```python
from build123d import *

# Parameters (mm, degrees)
BOSS_EXTRUDE1_DEPTH = 2
BOSS_EXTRUDE2_DEPTH = 20
FILLET1_R           = 5
CHAMFER1_SIZE       = 3.5
CHAMFER1_SIZE2      = 7.505774222


with BuildPart() as part:
    # Sketch1 → Boss-Extrude1 (new body)
    with BuildSketch(Plane(origin=(0, 0, 0), x_dir=(1, 0, 0), z_dir=(0, 1, 0))):
        with BuildLine():
            ThreePointArc((58.25, 100.891959541), (30.152418754, 112.530358763), (0, 116.5))
            Line((0, 116.5), (0, 105.5))
            ThreePointArc((0, 105.5), (27.305409258, 101.905174673), (52.75, 91.365680099))
            Line((52.75, 91.365680099), (58.25, 100.891959541))
        make_face()
    extrude(amount=BOSS_EXTRUDE1_DEPTH)

    # Sketch1<3> → Boss-Extrude2 (add)
    with BuildSketch(Plane(origin=(0, 0, 0), x_dir=(1, 0, 0), z_dir=(0, 1, 0))):
        with BuildLine():
            ThreePointArc((52.75, 91.365680099), (27.305409258, 101.905174673), (0, 105.5))
            Line((0, 105.5), (0, 101.5))
            ThreePointArc((0, 101.5), (26.270133078, 98.041471368), (50.75, 87.901578484))
            Line((50.75, 87.901578484), (52.75, 91.365680099))
        make_face()
    extrude(amount=BOSS_EXTRUDE2_DEPTH)

    # Fillet1
    fillet1_edges = [part.edges().sort_by_distance(p)[0] for p in [
        (27.305409258, 2, -101.905174673),
    ]]
    fillet(fillet1_edges, radius=FILLET1_R)

    # Chamfer1
    chamfer1_edges = [part.edges().sort_by_distance(p)[0] for p in [
        (27.305409258, 20, -101.905174673),
    ]]
    chamfer1_side = [part.faces().sort_by_distance(p)[0] for p in [
        (26.486113557, 20, -98.847521491),
    ]]
    chamfer(chamfer1_edges, length=CHAMFER1_SIZE, length2=CHAMFER1_SIZE2, reference=chamfer1_side[0])


solid = part.part
```
Geometry: final body of the model. Coordinates: model frame, mm. A direction names the side the tool comes from. Coordinates: 2 decimals unless noted, no trailing zeros. Loops run counter-clockwise (first coordinate to the right, second up) from the corner with the lowest first, then second, coordinate; pieces in that order, holes last. Notation, with made-up numbers: (88.5, 67) -> (110.5, 67) arc R38 ccw to (110.5, 106) -> close; hole circle Ø9 at (77.25, 66.25). An arc over 180 degrees is marked (long way). Use a Markdown table: item, result. Add a question column.
(1) Access query for faces 1 (the flat face through (29, 2, -108)), 2 (the flat face through (29, 0, -106)). Directions: +Z, -Z, +X, -X, +Y, -Y. A direction counts if a zero-diameter tool reaches every point of the face in a straight line with its end or side. Return the directions, or none.
(2) Section query C-C, the plane y = 18.5. Return loops of the section in (x, z).
(3) Section query A-A, the plane y = 10. Return loops of the section in (x, z).
(4) Section query B-B, the plane y = 2.75. Return loops of the section in (x, z), plus the area to 3 significant figures.
(5) Line query: line 1 along Y through (x, z) = (49, -104.5); line 2 along Z through (x, y) = (49, 18.5); line 3 along Z through (x, y) = (39, 18). Output: solid intervals per line, ascending.
(6) Pin query (flat end, axial travel): pin 1 Ø4 at (y, z) = (14.5, -97.5) entering from +X; pin 2 Ø10.5 at (x, z) = (14.5, -111.5) entering from +Y; pin 3 Ø4 at (y, z) = (13.5, -91.5) entering from -X. Return the tip coordinate at first contact, or that it passes through.
Answer:
| question | item | result |
|---|---|---|
| 1 | face 1 | -Z, +X, +Y |
| 1 | face 2 | +Z, -Z, +X, -X, -Y |
| 2 | outline | (0, -102.7) arc R102.7 ccw to (51.35, -88.94) -> (50.75, -87.9) arc R101.5 cw to (0, -101.5) -> close |
| 3 | outline | (0, -105.5) arc R105.5 ccw to (52.75, -91.37) -> (50.75, -87.9) arc R101.5 cw to (0, -101.5) -> close |
| 4 | outline | (0, -107.87) arc R107.87 ccw to (53.93, -93.41) -> (50.75, -87.9) arc R101.5 cw to (0, -101.5) -> close |
| 4 | area | 349 mm^2 |
| 5 | line 1 | y = 0 to 2 |
| 5 | line 2 | z = -90.26 to -88.89 |
| 5 | line 3 | z = -95.26 to -93.71 |
| 6 | pin 1 | stops at x = 43.13 |
| 6 | pin 2 | stops at y = 3.25 |
| 6 | pin 3 | stops at x = 39.5 |
